```python
from build123d import *

# Parameters (mm, degrees)
ESBO_O1_W                = 100
ESBO_O1_H                = 100
RESSALTO_EXTRUS_O1_DEPTH = 100
CORTE_EXTRUS_O1_REACH    = 152
ESBO_O2_R                = 4
ESBO_O3_R                = 7
ESBO_O3_R_2              = 1.7
CORTE_EXTRUS_O2_DEPTH    = 10


with BuildPart() as part:
    # Esboço1 → Ressalto-extrusão1 (new body)
    with BuildSketch(Plane.XY):
        Rectangle(ESBO_O1_W, ESBO_O1_H)
    extrude(amount=RESSALTO_EXTRUS_O1_DEPTH)

    # Esboço2 → Corte-extrusão1 (cut, up to next)
    with BuildSketch(Plane(origin=(50, 0, 0), x_dir=(0, 0, -1), z_dir=(1, 0, 0)), mode=Mode.PRIVATE) as corte_extrus_o1_sk1:
        with Locations((-40, 0)):
            Circle(ESBO_O2_R)
    corte_extrus_o1_tool1 = extrude(corte_extrus_o1_sk1.sketch, amount=-CORTE_EXTRUS_O1_REACH, mode=Mode.PRIVATE) & part.part
    # Esboço2 → Corte-extrusão1 (cut, up to next)
    with BuildSketch(Plane(origin=(50, 0, 0), x_dir=(0, 0, -1), z_dir=(1, 0, 0)), mode=Mode.PRIVATE) as corte_extrus_o1_sk2:
        with Locations((-60, 0)):
            Circle(ESBO_O2_R)
    corte_extrus_o1_tool2 = extrude(corte_extrus_o1_sk2.sketch, amount=-CORTE_EXTRUS_O1_REACH, mode=Mode.PRIVATE) & part.part
    add(corte_extrus_o1_tool1.solids().sort_by_distance((50, 0, 40))[0], mode=Mode.SUBTRACT)
    add(corte_extrus_o1_tool2.solids().sort_by_distance((50, 0, 60))[0], mode=Mode.SUBTRACT)

    # Esboço3 → Corte-extrusão2 (cut)
    with BuildSketch(Plane(origin=(0, -50, 0), x_dir=(-1, 0, 0), z_dir=(0, -1, 0))):
        with Locations(Location((0, -50, 0), (0, 0, 180))):
            Circle(ESBO_O3_R)
        with Locations(Location((0, -25, 0), (0, 0, 180))):
            Circle(ESBO_O3_R_2)
        with Locations(Location((21.650635095, -62.5, 0), (0, 0, 180))):
            Circle(ESBO_O3_R_2)
        with Locations(Location((-21.650635095, -62.5, 0), (0, 0, 180))):
            Circle(ESBO_O3_R_2)
    extrude(amount=-CORTE_EXTRUS_O2_DEPTH, mode=Mode.SUBTRACT)


solid = part.part
```
Verification items for the finished model (mm, model axes). A direction names the side the tool comes from. Give positions to 0.01 mm unless a question says otherwise; leave off trailing zeros. Order: outer loops, then holes, each group sorted by start corner. A loop starts at its lowest first (then second) coordinate and runs counter-clockwise, first axis right, second up. Notation, with made-up numbers: M -4,-13 L 50,-13 A29 cw 50,11 Z; hole C 53.25,-6.75 d6. An arc over 180 degrees is marked long. Return JSON: item names as keys, results as strings. Group by question number.
1) Go/stop test with flat-tipped pins: pin 1 Ø2.5 at (x, z) = (-21.65, 62.5) entering from -Y; pin 2 Ø5 at (x, y) = (-9, 17) entering from -Z. Record where each tip stops, or that it passes through.
2) Scan lines: line 1 (Z direction, x = 0, y = -47); line 2 (Y direction, x = 18, z = 40); line 3 (Z direction, x = 21, y = -44). Record each from-to range of solid material in increasing order.
3) Section check A-A on y = 0. Record the cut outline in (x, z).
4) Section check D-D on y = -43.5. Record the cut outline in (x, z), and give its area (3 significant figures).
5) Access from +Z, -Z, +X, -X, +Y, -Y to the whole of each face (thin tool, end or side, straight path). Record for faces 1 (the face through (-1, -50, 38)), 2 (the face through (-0.91, -45.07, 56.94)).
6) Mould release check, pull along Y, two halves, no side actions. Record for faces 3 (the face through (0.7, 1.201, 56.185)), 4 (the face through (-1, 1, 0)), 5 (the face through (-22, -40, 63)): pulls with the +Y half, pulls with the -Y half, needs draft (parallel to the pull), parting line crosses it, or undercut.
7) Section check B-B on x = 0. Record the cut outline in (y, z).
8) Section check C-C on z = 40. Record the cut outline in (x, y), and give its area (3 significant figures).
Answer block:
{
 "1": {"pin 1": "stops at y = -40", "pin 2": "stops at z = 0"},
 "2": {"line 1": "z = 0 to 23.3, 26.7 to 43, 57 to 100", "line 2": "y = -50 to -4, 4 to 50", "line 3": "z = 0 to 60.93, 64.07 to 100"},
 "3": {"outline": "M -50,0 L 50,0 L 50,36 L -50,36 Z; M -50,44 L 50,44 L 50,56 L -50,56 Z; M -50,64 L 50,64 L 50,100 L -50,100 Z"},
 "4": {"outline": "M -50,0 L 50,0 L 50,100 L -50,100 Z; hole C -21.65,62.5 d3.4; hole C 0,50 d14; hole C 0,25 d3.4; hole C 21.65,62.5 d3.4", "area": "9,820 mm^2"},
 "5": {"face 1": "+Z, -Z, +X, -X, -Y", "face 2": "-Y"},
 "6": {"face 3": "undercut", "face 4": "needs draft", "face 5": "pulls with the -Y half"},
 "7": {"outline": "M -50,0 L 50,0 L 50,100 L -50,100 L -50,57 L -40,57 L -40,43 L -50,43 L -50,26.7 L -40,26.7 L -40,23.3 L -50,23.3 Z; hole C 0,40 d8; hole C 0,60 d8"},
 "8": {"outline": "M -50,-50 L 50,-50 L 50,-4 L -50,-4 Z; M -50,4 L 50,4 L 50,50 L -50,50 Z", "area": "9,200 mm^2"}
}
